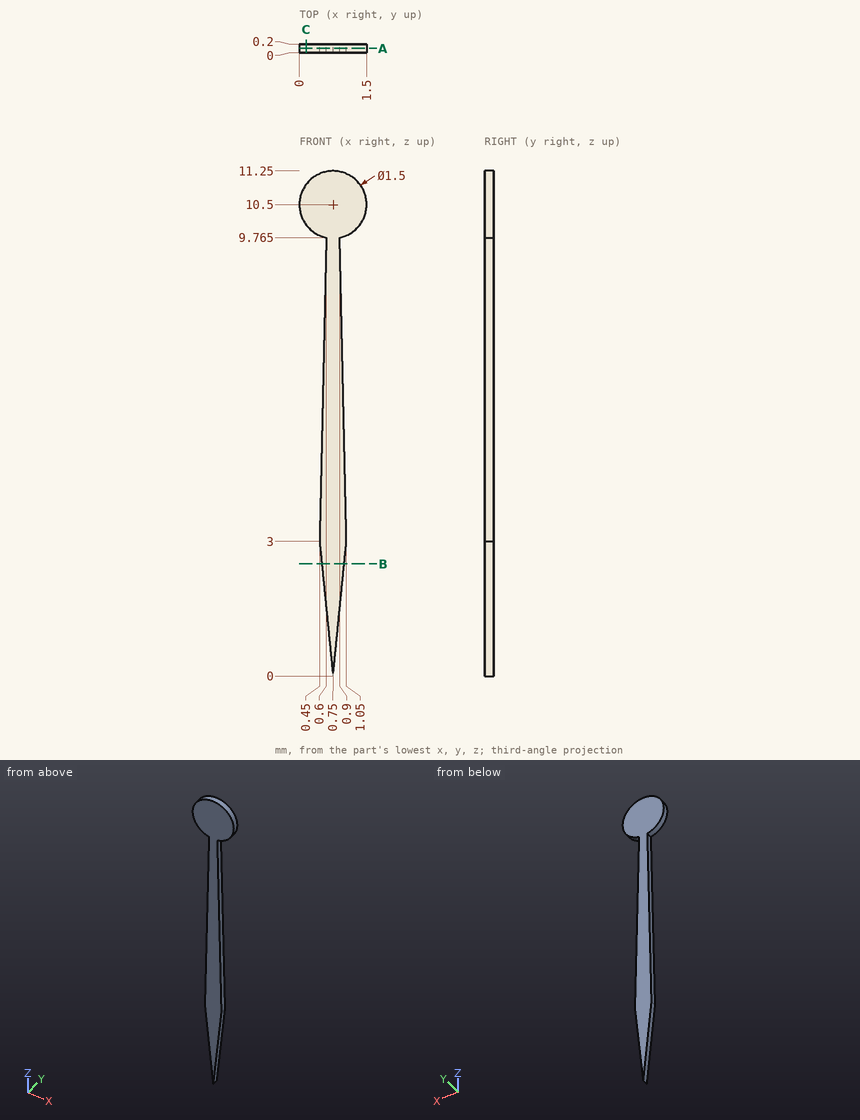
Check sheet for the drawn part. Datum: minimum x, y, z corner. Units: mm. Give positions to 0.01 mm unless a question says otherwise; leave off trailing zeros. Loops run counter-clockwise (first coordinate to the right, second up) from the corner with the lowest first, then second, coordinate; pieces in that order, holes last.
1) Thickness scan on line 1 along X through (y, z) = (0.1, 1); line 2 along X through (y, z) = (0.1, 5); line 3 along Z through (x, y) = (1.4, 0.05) (1 decimal). Record the ranges inside material, lowest first.
2) Sectioned sample at B-B, the plane z = 2.5. Enter the section's corners in (x, y).
3) Sectioned sample at A-A, the plane y = 0.1. Enter the section's corners in (x, z) (3 decimals).
4) Sectioned sample at C-C, the plane x = 0.15. Enter the section's corners in (y, z).
Answers:
1. line 1: x = 0.65 to 0.85
1. line 2: x = 0.49 to 1.01
1. line 3: z = 10.1 to 10.9
2. outline: (0.5, 0) - (1, 0) - (1, 0.2) - (0.5, 0.2) - close
3. outline: (0.45, 3) - (0.75, 0) - (1.05, 3) - (0.9, 9.765) arc R0.75 ccw (long way) to (0.6, 9.765) - close
4. outline: (0, 10.05) - (0.2, 10.05) - (0.2, 10.95) - (0, 10.95) - close
